```python
from build123d import *

# Parameters (mm, degrees)
SKETCH_1_R      = 1.000000438
EXTRUDE_1_DEPTH = 3


with BuildPart() as part:
    # 草图1 → 凸台-拉伸1 (new body)
    with BuildSketch(Plane.XY):
        with BuildLine():
            Line((60.073949397, -2.000000095), (57.073947042, -4.00000019))
            Line((57.073947042, -4.00000019), (7.913790643, -7.376036607))
            Line((7.913790643, -7.376036607), (6.708230358, -6.708230358))
            Line((6.708230358, -6.708230358), (6.916883867, -7.454637904))
            Line((6.916883867, -7.454637904), (0.500000024, -7.960577495))
            Line((0.500000024, -7.960577495), (0, -7.000000216))
            Line((0, -7.000000216), (-0.500000024, -7.934173569))
            ThreePointArc((-0.500000024, -7.934173569), (-3.067102082, -7.398918018), (-5.260177422, -5.961235147))
            Line((-5.260177422, -5.961235147), (-4.949747585, -4.949747585))
            Line((-4.949747585, -4.949747585), (-5.961235147, -5.260177422))
            ThreePointArc((-5.961235147, -5.260177422), (-7.966566676, 0), (-5.961235147, 5.260177422))
            Line((-5.961235147, 5.260177422), (-4.949747585, 4.949747585))
            Line((-4.949747585, 4.949747585), (-5.260177422, 5.961235147))
            ThreePointArc((-5.260177422, 5.961235147), (-3.067102082, 7.398918018), (-0.500000024, 7.934173569))
            Line((-0.500000024, 7.934173569), (0, 7.000000216))
            Line((0, 7.000000216), (0.500000024, 7.960577495))
            Line((0.500000024, 7.960577495), (6.916883867, 7.454637904))
            Line((6.916883867, 7.454637904), (6.708230358, 6.708230358))
            Line((6.708230358, 6.708230358), (7.913790643, 7.376036607))
            Line((7.913790643, 7.376036607), (57.073947042, 4.00000019))
            Line((57.073947042, 4.00000019), (60.073949397, 2.000000095))
            Line((60.073949397, 2.000000095), (57.573948056, 2.000000095))
            ThreePointArc((57.573948056, 2.000000095), (56.720394687, 2.35355404), (57.073947042, 1.500000013))
            Line((57.073947042, 1.500000013), (57.073947042, -1.500000013))
            ThreePointArc((57.073947042, -1.500000013), (56.720394687, -2.35355404), (57.573948055, -2.000000095))
            Line((57.573948055, -2.000000095), (60.073949397, -2.000000095))
        make_face()
        with Locations((25.073947659, -3.992e-06)):
            Circle(SKETCH_1_R, mode=Mode.SUBTRACT)
        with BuildLine():
            Line((42.073946446, 2.116752788), (51.073949784, 2.000000095))
            Line((51.073949784, 2.000000095), (53.5739474, 2.000000095))
            ThreePointArc((53.5739474, 2.000000095), (54.427500768, 2.35355404), (54.073948413, 1.500000013))
            Line((54.073948413, 1.500000013), (54.073948413, -1.500000013))
            ThreePointArc((54.073948413, -1.500000013), (54.427500768, -2.35355404), (53.5739474, -2.000000095))
            Line((53.5739474, -2.000000095), (51.073949784, -2.000000095))
            Line((51.073949784, -2.000000095), (42.073946446, -2.116752788))
            Line((42.073946446, -2.116752788), (42.073946446, 2.116752788))
        make_face(mode=Mode.SUBTRACT)
        with BuildLine():
            Line((27.573948726, 2.000000095), (28.823947534, 2.000000095))
            Line((28.823947534, 2.000000095), (30.073948204, 2.9390899))
            Line((30.073948204, 2.9390899), (39.073947817, 2.322337125))
            Line((39.073947817, 2.322337125), (39.073947817, -2.322337125))
            Line((39.073947817, -2.322337125), (30.073948204, -2.9390899))
            Line((30.073948204, -2.9390899), (28.823947534, -2.000000095))
            Line((28.823947534, -2.000000095), (27.573948726, -2.000000095))
            ThreePointArc((27.573948726, -2.000000095), (26.720395358, -2.35355404), (27.073947713, -1.500000013))
            Line((27.073947713, -1.500000013), (27.073947713, 1.500000013))
            ThreePointArc((27.073947713, 1.500000013), (26.720395358, 2.35355404), (27.573948726, 2.000000095))
        make_face(mode=Mode.SUBTRACT)
        with BuildLine():
            Line((-4.00000019, 0.500000024), (-1.980265602, 0.500000024))
            ThreePointArc((-1.980265602, 0.500000024), (0, 2.052275233), (1.980265603, 0.500000024))
            Line((1.980265603, 0.500000024), (6.000000052, 0.500000024))
            Line((6.000000052, 0.500000024), (6.000000052, -0.500000024))
            Line((6.000000052, -0.500000024), (1.980265602, -0.500000024))
            ThreePointArc((1.980265602, -0.500000024), (0, -2.052275233), (-1.980265603, -0.500000024))
            Line((-1.980265603, -0.500000024), (-4.00000019, -0.500000024))
            Line((-4.00000019, -0.500000024), (-4.00000019, 0.500000024))
        make_face(mode=Mode.SUBTRACT)
        Polygon((12.073948048, -4.172595218), (23.07394892, -3.350258339), (23.07394892, 3.350258339), (12.073948048, 4.172595218), align=None, mode=Mode.SUBTRACT)
    extrude(amount=EXTRUDE_1_DEPTH)


solid = part.part
```
The model under review builds one solid part; all positions refer to its coordinate system, in mm. A direction names the side the tool comes from. Coordinates: 2 decimals unless noted, no trailing zeros. Write each loop counter-clockwise with the first axis right and the second up, starting at its lowest first coordinate (ties: lowest second). Pieces come first, ordered by that corner, then holes. Notation, with made-up numbers: (-14, 83) - (0, 83) arc R24 cw to (0, 97) - close; hole circle Ø11 at (21, 71). An arc over 180 degrees is marked (long way). Answer in a Markdown table with one row per item. Add a question column.
Q1. Clearance check with flat-ended pins moving along their axes: pin 1 (6 mm diameter, centred on x = 26, y = -5.5, fed in from -Z); pin 2 (1.5 mm diameter, centred on y = -0.5, z = 1.5, fed in from +X); pin 3 (1.2 mm diameter, centred on x = 53, z = 1.5, fed in from +Y); pin 4 (1.5 mm diameter, centred on x = 23, z = 2.5, fed in from -Y). State where each tip first meets the part, or that it passes through.
Q2. Consider section C-C on x = 52.5. Give the boundary of the cut face in (y, z).
Q3. Consider section A-A on x = 37.5. Give the boundary of the cut face in (y, z).
Q4. Draft analysis for pull direction Y (two halves, no side actions). For faces 1 (the face through (19, -5, 0)), 2 (the face through (3.66, 7.71, 1.48)), 3 (the face through (4, 0.5, 1)), state which applies: +Y half, -Y half, draft (parallel to the pull), parting line (faces both ways), or undercut.
Q5. To check wall thickness, follow line 1 along Y through (x, z) = (16, 1.45); line 2 along Y through (x, z) = (28.5, 2); line 3 along X through (y, z) = (3.25, 1.7). State the ranges of each line that lie inside material, in increasing order. Write a range as from..to.
Q6. For faces 4 (the face through (32.838, -5.664, 1.479)), 5 (the face through (59, -2, 1)), 6 (the face through (12.074, 0, 1)), list the 3-axis set-ups (+Z, -Z, +X, -X, +Y, -Y) from which the entire face can be reached by the end or side of a thin tool; tool diameter is ignored.
Q7. Consider section B-B on z = 1. Give the number of separate pieces and of enclosed holes in the cut face, then the cut area to 3 significant figures.
Answers below:
| question | item | result |
|---|---|---|
| 1 | pin 1 | z = 0 |
| 1 | pin 2 | x = 57.07 |
| 1 | pin 3 | y = 4.32 |
| 1 | pin 4 | y = -6.39 |
| 2 | outline | (-4.31, 0) - (-2, 0) - (-2, 3) - (-4.31, 3) - close; (2, 0) - (4.31, 0) - (4.31, 3) - (2, 3) - close |
| 3 | outline | (-5.34, 0) - (-2.43, 0) - (-2.43, 3) - (-5.34, 3) - close; (2.43, 0) - (5.34, 0) - (5.34, 3) - (2.43, 3) - close |
| 4 | face 1 | draft |
| 4 | face 2 | +Y half |
| 4 | face 3 | undercut |
| 5 | line 1 | -6.82..-3.88, 3.88..6.82 |
| 5 | line 2 | -5.96..-2, 2..5.96 |
| 5 | line 3 | -7.27..12.07, 23.07..58.2 |
| 6 | face 4 | +Z, -Z, +X, -Y |
| 6 | face 5 | +Z, -Z, +X |
| 6 | face 6 | +Z, -Z |
| 7 | separate pieces | 1 |
| 7 | enclosed holes | 5 |
| 7 | area | 566 mm² |
